from build123d import *

# Parameters (mm, degrees)
SKETCH1_W           = 102
SKETCH1_H           = 85
BOSS_EXTRUDE1_DEPTH = 7.5
SKETCH2_W           = 98
SKETCH2_H           = 81
CUT_EXTRUDE1_DEPTH  = 5.5
SKETCH3_R           = 5
BOSS_EXTRUDE2_DEPTH = 4
SKETCH3_3_R         = 5
BOSS_EXTRUDE3_DEPTH = 5
SKETCH4_R           = 3
CUT_EXTRUDE3_DEPTH  = 3
SKETCH5_R           = 1.6
CUT_EXTRUDE4_DEPTH  = 7.5
SKETCH6_W           = 14.3
SKETCH6_H           = 26
CUT_EXTRUDE5_DEPTH  = 10
CHAMFER1_SIZE       = 1.5
CHAMFER2_SIZE       = 1.5
CHAMFER3_SIZE       = 1.5
CHAMFER4_SIZE       = 1.5
SKETCH7_R           = 3.25
CUT_EXTRUDE6_DEPTH  = 10
FILLET2_R           = 5
FILLET3_SIZE        = 5
FILLET4_R           = 5
FILLET5_SIZE        = 5
FILLET6_SIZE        = 5
FILLET7_SIZE        = 5
FILLET8_SIZE        = 5
FILLET9_SIZE        = 5
SKETCH8_R           = 3
CUT_EXTRUDE7_DEPTH  = 3


with BuildPart() as part:
    # Sketch1 → Boss-Extrude1 (new body)
    with BuildSketch(Plane(origin=(0, 0, 0), x_dir=(1, 0, 0), z_dir=(0, 1, 0))):
        Rectangle(SKETCH1_W, SKETCH1_H)
    extrude(amount=BOSS_EXTRUDE1_DEPTH)

    # Sketch2 → Cut-Extrude1 (cut)
    with BuildSketch(Plane(origin=(0, 7.5, 0), x_dir=(1, 0, 0), z_dir=(0, 1, 0))):
        Rectangle(SKETCH2_W, SKETCH2_H)
    extrude(amount=-CUT_EXTRUDE1_DEPTH, mode=Mode.SUBTRACT)



with BuildPart() as body_2:
    # Sketch3 → Boss-Extrude2 (new body)
    with BuildSketch(Plane(origin=(0, 0, 0), x_dir=(-1, 0, 0), z_dir=(0, -1, 0))):
        with Locations(Location((43, -34.5, 0), (0, 0, 90))):
            Circle(SKETCH3_R)
    extrude(amount=-BOSS_EXTRUDE2_DEPTH)


with BuildPart() as part_1:
    add(part.part)

    add(body_2.part)  # Boss-Extrude3 merges body 2
    # Sketch3<3> → Boss-Extrude3 (add)
    with BuildSketch(Plane(origin=(0, 0, 0), x_dir=(-1, 0, 0), z_dir=(0, -1, 0))):
        with Locations(Location((43, -34.5, 0), (0, 0, 90))):
            Circle(SKETCH3_3_R)
        with Locations(Location((-43, -34.5, 0), (0, 0, 90))):
            Circle(SKETCH3_3_R)
        with Locations(Location((43, 34.5, 0), (0, 0, 90))):
            Circle(SKETCH3_3_R)
        with Locations(Location((-43, 34.5, 0), (0, 0, 90))):
            Circle(SKETCH3_3_R)
    extrude(amount=-BOSS_EXTRUDE3_DEPTH)

    # Sketch4 → Cut-Extrude3 (cut)
    with BuildSketch(Plane.XZ):
        with Locations(Location((-43, 34.5, 0), (0, 0, 270))):
            Circle(SKETCH4_R)
        with Locations(Location((43, 34.5, 0), (0, 0, 270))):
            Circle(SKETCH4_R)
        with Locations(Location((-43, -34.5, 0), (0, 0, 270))):
            Circle(SKETCH4_R)
        with Locations(Location((43, -34.5, 0), (0, 0, 270))):
            Circle(SKETCH4_R)
    extrude(amount=-CUT_EXTRUDE3_DEPTH, mode=Mode.SUBTRACT)

    # Sketch5 → Cut-Extrude4 (cut)
    with BuildSketch(Plane.XZ):
        with Locations(Location((-43, 34.5, 0), (0, 0, 270))):
            Circle(SKETCH5_R)
        with Locations(Location((43, 34.5, 0), (0, 0, 270))):
            Circle(SKETCH5_R)
        with Locations(Location((43, -34.5, 0), (0, 0, 270))):
            Circle(SKETCH5_R)
        with Locations(Location((-43, -34.5, 0), (0, 0, 270))):
            Circle(SKETCH5_R)
    extrude(amount=-CUT_EXTRUDE4_DEPTH, mode=Mode.SUBTRACT)

    # Sketch6 → Cut-Extrude5 (cut)
    with BuildSketch(Plane.XZ):
        with Locations((25.35, 0)):
            Rectangle(SKETCH6_W, SKETCH6_H)
    extrude(amount=-CUT_EXTRUDE5_DEPTH, mode=Mode.SUBTRACT)

    # Chamfer1
    chamfer1_edges = [part_1.edges().sort_by_distance(p)[0] for p in [
        (25.35, 0, 13),
    ]]
    chamfer(chamfer1_edges, length=CHAMFER1_SIZE)

    # Chamfer2
    chamfer2_edges = [part_1.edges().sort_by_distance(p)[0] for p in [
        (18.2, 0, 0.75),
    ]]
    chamfer(chamfer2_edges, length=CHAMFER2_SIZE)

    # Chamfer3
    chamfer3_edges = [part_1.edges().sort_by_distance(p)[0] for p in [
        (32.5, 0, 0.75),
    ]]
    chamfer(chamfer3_edges, length=CHAMFER3_SIZE)

    # Chamfer4
    chamfer4_edges = [part_1.edges().sort_by_distance(p)[0] for p in [
        (25.35, 0, -13),
    ]]
    chamfer(chamfer4_edges, length=CHAMFER4_SIZE)

    # Sketch7 → Cut-Extrude6 (cut)
    with BuildSketch(Plane(origin=(0, 0, 0), x_dir=(-1, 0, 0), z_dir=(0, -1, 0))):
        with Locations(Location((-39.2, -26.7, 0), (0, 0, 90))):
            Circle(SKETCH7_R)
    extrude(amount=-CUT_EXTRUDE6_DEPTH, mode=Mode.SUBTRACT)

    # Fillet2
    fillet2_edges = [part_1.edges().sort_by_distance(p)[0] for p in [
        (51, 3.75, 42.5),
    ]]
    fillet(fillet2_edges, radius=FILLET2_R)

    # Fillet3
    # a fillet whose section is not a circle: 5 mm, written as the material it takes off along each edge
    with BuildSketch(Plane(origin=(51, -12.5, -42.5), x_dir=(0, 0, 1), z_dir=(0, 1, 0))) as fillet3_piece_1:
        with BuildLine():
            Bezier((FILLET3_SIZE, 0), (0, 0), (0, -FILLET3_SIZE), weights=[1, 1, 1])
            Line((0, -FILLET3_SIZE), (0, 0))
            Line((0, 0), (FILLET3_SIZE, 0))
        make_face()
    extrude(amount=32.5, mode=Mode.SUBTRACT)

    # Fillet4
    fillet4_edges = [part_1.edges().sort_by_distance(p)[0] for p in [
        (-51, 3.75, 42.5),
    ]]
    fillet(fillet4_edges, radius=FILLET4_R)

    # Fillet5
    # a fillet whose section is not a circle: 5 mm, written as the material it takes off along each edge
    with BuildSketch(Plane(origin=(-51, -12.5, -42.5), x_dir=(0, 0, 1), z_dir=(0, 1, 0))) as fillet5_piece_1:
        with BuildLine():
            add(Edge.make_bspline([(FILLET5_SIZE, 0), (FILLET5_SIZE * 0.831801948466, 0), (FILLET5_SIZE * 0.663603896932, 0), (FILLET5_SIZE * 0.292893218813, FILLET5_SIZE * 0.0716919198361), (FILLET5_SIZE * 0.0716919198361, FILLET5_SIZE * 0.292893218813), (0, FILLET5_SIZE * 0.663603896932), (0, FILLET5_SIZE * 0.831801948466), (0, FILLET5_SIZE)], knots=[0, 0, 0, 0, 0, 0, 0.5, 0.5, 1, 1, 1, 1, 1, 1], degree=5))
            Line((0, FILLET5_SIZE), (0, 0))
            Line((0, 0), (FILLET5_SIZE, 0))
        make_face()
    extrude(amount=32.5, mode=Mode.SUBTRACT)

    # Fillet6
    # a fillet whose section is not a circle: 5 mm, written as the material it adds along each edge
    with BuildSketch(Plane(origin=(49, 7.5, -40.5), x_dir=(-1, 0, 0), z_dir=(0, -1, 0))) as fillet6_piece_1:
        with BuildLine():
            Bezier((FILLET6_SIZE, 0), (0, 0), (0, -FILLET6_SIZE), weights=[1, 1, 1])
            Line((0, -FILLET6_SIZE), (0, 0))
            Line((0, 0), (FILLET6_SIZE, 0))
        make_face()
    extrude(amount=5.5)

    # Fillet7
    # a fillet whose section is not a circle: 5 mm, written as the material it adds along each edge
    with BuildSketch(Plane(origin=(49, 7.5, 40.5), x_dir=(0, 0, -1), z_dir=(0, -1, 0))) as fillet7_piece_1:
        with BuildLine():
            Bezier((FILLET7_SIZE, 0), (0, 0), (0, -FILLET7_SIZE), weights=[1, 1, 1])
            Line((0, -FILLET7_SIZE), (0, 0))
            Line((0, 0), (FILLET7_SIZE, 0))
        make_face()
    extrude(amount=5.5)

    # Fillet8
    # a fillet whose section is not a circle: 5 mm, written as the material it adds along each edge
    with BuildSketch(Plane(origin=(-49, 7.5, 40.5), x_dir=(1, 0, 0), z_dir=(0, -1, 0))) as fillet8_piece_1:
        with BuildLine():
            Bezier((FILLET8_SIZE, 0), (0, 0), (0, -FILLET8_SIZE), weights=[1, 1, 1])
            Line((0, -FILLET8_SIZE), (0, 0))
            Line((0, 0), (FILLET8_SIZE, 0))
        make_face()
    extrude(amount=5.5)

    # Fillet9
    # a fillet whose section is not a circle: 5 mm, written as the material it adds along each edge
    with BuildSketch(Plane(origin=(-49, 7.5, -40.5), x_dir=(0, 0, 1), z_dir=(0, -1, 0))) as fillet9_piece_1_section:
        with BuildLine():
            Bezier((FILLET9_SIZE, 0), (0, 0), (0, -FILLET9_SIZE), weights=[1, 1, 1])
            Line((0, -FILLET9_SIZE), (0, 0))
            Line((0, 0), (FILLET9_SIZE, 0))
        make_face()
    fillet9_piece_1 = extrude(amount=18, mode=Mode.PRIVATE)
    fillet9_piece_1 = split(fillet9_piece_1, bisect_by=Plane(origin=(-49, 0, -40.5), z_dir=(0, 1, 0)), keep=Keep.TOP, mode=Mode.PRIVATE)
    add(fillet9_piece_1)

    # Sketch8 → Cut-Extrude7 (cut)
    with BuildSketch(Plane.XZ):
        with Locations(Location((-3.9, -12.35, 0), (0, 0, 270))):
            Circle(SKETCH8_R)
        with Locations(Location((-3.9, -0.05, 0), (0, 0, 270))):
            Circle(SKETCH8_R)
        with Locations(Location((-3.9, 12.35, 0), (0, 0, 270))):
            Circle(SKETCH8_R)
    extrude(amount=-CUT_EXTRUDE7_DEPTH, mode=Mode.SUBTRACT)


solid = part_1.part
Design review of the part built by this model. Coordinates are the model's own, in mm. A direction names the side the tool comes from. Give positions to 0.01 mm unless a question says otherwise; leave off trailing zeros. Loops run counter-clockwise (first coordinate to the right, second up) from the corner with the lowest first, then second, coordinate; pieces in that order, holes last. Notation, with made-up numbers: (47.25, -7.5) - (57.25, -7.5) arc R22 ccw to (57.25, 11.5) - close; hole circle Ø7 at (64.5, 24.25). An arc over 180 degrees is marked (long way). Write item = value, one per line.
1) Draft analysis for pull direction X (two halves, no side actions). For faces 1 (the face through (1, 0, 1)), 2 (the face through (-44, 3, -36)), 3 (the face through (-51, 4, 1)), 4 (the face through (-43.97, 3.99, 35.77)), state which applies: +X half, -X half, draft (parallel to the pull), parting line (faces both ways), or undercut.
Result sheet:
face_1 = draft
face_2 = undercut
face_3 = -X half
face_4 = undercut
2) Take a section at A-A on z = 26.7. State the section outline as (x, y) points, and give its area (3 significant figures).
Result sheet:
outline = (-51, 0) - (35.95, 0) - (35.95, 2) - (-49, 2) - (-49, 7.5) - (-51, 7.5) - close; (42.45, 0) - (51, 0) - (51, 7.5) - (49, 7.5) - (49, 2) - (42.45, 2) - close
area = 213 mm2
3) To check wall thickness, follow line 1 (X direction, y = 2.25, z = -34.5); line 2 (X direction, y = 1.65, z = -34.5); line 3 (X direction, y = 3.8, z = -34.5). State the ranges of each line that lie inside material, in increasing order.
Result sheet:
line_1 = -51 to -49, -48 to -46, -40 to -38, 38 to 40, 46 to 48, 49 to 51
line_2 = -51 to -46, -40 to 40, 46 to 51
line_3 = -51 to -49, -48 to -44.6, -41.4 to -38, 38 to 41.4, 44.6 to 48, 49 to 51
4) Clearance check with flat-ended pins moving along their axes: pin 1 Ø1 at (x, z) = (-24, -19) entering from +Y; pin 2 Ø3.5 at (x, z) = (43, 34.5) entering from +Y; pin 3 Ø3.5 at (x, z) = (-43, 34.5) entering from -Y. State where each tip first meets the part, or that it passes through.
Result sheet:
pin_1 = 2
pin_2 = 5
pin_3 = 3
5) Tool access review of faces 5 (the face through (-42, 5, -33)), 6 (the face through (42.422, 0.986, 27.123)), 7 (the face through (42, 3, 33)): name each direction out of +Z, -Z, +X, -X, +Y, -Y from which nothing blocks a thin tool from reaching the whole face with its end or side.
Result sheet:
face_5 = +Y
face_6 = +Y, -Y
face_7 = -Y
6) Take a section at C-C on z = -0.05. State the section outline as (x, y) points, and give its area (3 significant figures).
Result sheet:
outline = (-51, 0) - (-6.9, 0) - (-6.9, 2) - (-49, 2) - (-49, 7.5) - (-51, 7.5) - close; (-0.9, 0) - (16.7, 0) - (18.2, 1.5) - (18.2, 2) - (-0.9, 2) - close; (32.5, 1.5) - (34, 0) - (51, 0) - (51, 7.5) - (49, 7.5) - (49, 2) - (32.5, 2) - close
area = 183 mm2
7) Take a section at B-B on x = -3.9. State the section outline as (y, z) points.
Result sheet:
outline = (0, -42.5) - (7.5, -42.5) - (7.5, -40.5) - (2, -40.5) - (2, -15.35) - (0, -15.35) - close; (0, -9.35) - (2, -9.35) - (2, -3.05) - (0, -3.05) - close; (0, 2.95) - (2, 2.95) - (2, 9.35) - (0, 9.35) - close; (0, 15.35) - (2, 15.35) - (2, 40.5) - (7.5, 40.5) - (7.5, 42.5) - (0, 42.5) - close
8) Take a section at D-D on x = 23. State the section outline as (y, z) points, and give its area (3 significant figures).
Result sheet:
outline = (0, -42.5) - (7.5, -42.5) - (7.5, -40.5) - (2, -40.5) - (2, -13) - (1.5, -13) - (0, -14.5) - close; (0, 14.5) - (1.5, 13) - (2, 13) - (2, 40.5) - (7.5, 40.5) - (7.5, 42.5) - (0, 42.5) - close
area = 138 mm2
